Design review of the part built by this model. Coordinates are the model's own, in mm. A direction names the side the tool comes from. Give positions to 0.01 mm unless a question says otherwise; leave off trailing zeros. Order: outer loops, then holes, each group sorted by start corner. A loop starts at its lowest first (then second) coordinate and runs counter-clockwise, first axis right, second up. Notation, with made-up numbers: (14, 44.5) -> (64, 44.5) arc R12 ccw to (64, 66.5) -> close; hole circle Ø6 at (-1, 68). An arc over 180 degrees is marked (long way). Use a Markdown table: item, result. Add a question column.
```python
from build123d import *

# Parameters (mm, degrees)
BOSS_EXTRUDE1_DEPTH              = 9.525
TAP_DRILL_FOR_M3X0_5_TAP1_D      = 2.5
TAP_DRILL_FOR_M3X0_5_TAP2_D      = 2.5
TAP_DRILL_FOR_M3X0_5_TAP3_REACH  = 42.274
TAP_DRILL_FOR_M3X0_5_TAP3_BORE_R = 1.25
M3_CLEARANCE_HOLE1_REACH         = 42.274
M3_CLEARANCE_HOLE1_BORE_R        = 1.6


with BuildPart() as part:
    # Sketch1 → Boss-Extrude1 (new body)
    with BuildSketch(Plane(origin=(0, 0, 0), x_dir=(1, 0, 0), z_dir=(0, 1, 0))):
        with BuildLine():
            Line((-17.5, 17.5), (-5, 17.5))
            Line((-5, 17.5), (5, 17.5))
            Line((5, 17.5), (17.5, 17.5))
            Line((17.5, 17.5), (17.5, -17.5))
            Line((17.5, -17.5), (5, -17.5))
            Line((5, -17.5), (5, -8.660254038))
            ThreePointArc((5, -8.660254038), (10, 0), (5, 8.660254038))
            ThreePointArc((5, 8.660254038), (0, 10), (-5, 8.660254038))
            ThreePointArc((-5, 8.660254038), (-10, 0), (-5, -8.660254038))
            Line((-5, -8.660254038), (-5, -17.5))
            Line((-5, -17.5), (-17.5, -17.5))
            Line((-17.5, -17.5), (-17.5, 17.5))
        make_face()
    extrude(amount=BOSS_EXTRUDE1_DEPTH)

    # Tap Drill for M3x0.5 Tap1 (through all)
    with Locations(Plane(origin=(0, 9.525, 0), x_dir=(1, 0, 0), z_dir=(0, 1, 0))):
        with Locations((-15, 0)):
            Hole(TAP_DRILL_FOR_M3X0_5_TAP1_D / 2)

    # Tap Drill for M3x0.5 Tap2 (through all)
    with Locations(Plane(origin=(0, 9.525, 0), x_dir=(1, 0, 0), z_dir=(0, 1, 0))):
        with Locations((15, 0)):
            Hole(TAP_DRILL_FOR_M3X0_5_TAP2_D / 2)

    # Tap Drill for M3x0.5 Tap3 bore → Tap Drill for M3x0.5 Tap3 (cut, up to next)
    with BuildSketch(Plane(origin=(17.5, 0, 0), x_dir=(0, 0, -1), z_dir=(1, 0, 0)), mode=Mode.PRIVATE) as tap_drill_for_m3x0_5_tap3_sk1:
        with Locations((13.08015, 4.7625)):
            Circle(TAP_DRILL_FOR_M3X0_5_TAP3_BORE_R)
    tap_drill_for_m3x0_5_tap3_tool1 = extrude(tap_drill_for_m3x0_5_tap3_sk1.sketch, amount=-TAP_DRILL_FOR_M3X0_5_TAP3_REACH, mode=Mode.PRIVATE) & part.part
    # Tap Drill for M3x0.5 Tap3 bore → Tap Drill for M3x0.5 Tap3 (cut, up to next)
    with BuildSketch(Plane(origin=(17.5, 0, 0), x_dir=(0, 0, -1), z_dir=(1, 0, 0)), mode=Mode.PRIVATE) as tap_drill_for_m3x0_5_tap3_sk2:
        with Locations((-13.08015, 4.7625)):
            Circle(TAP_DRILL_FOR_M3X0_5_TAP3_BORE_R)
    tap_drill_for_m3x0_5_tap3_tool2 = extrude(tap_drill_for_m3x0_5_tap3_sk2.sketch, amount=-TAP_DRILL_FOR_M3X0_5_TAP3_REACH, mode=Mode.PRIVATE) & part.part
    add(tap_drill_for_m3x0_5_tap3_tool1.solids().sort_by_distance((17.5, 4.7625, -13.08015))[0], mode=Mode.SUBTRACT)
    add(tap_drill_for_m3x0_5_tap3_tool2.solids().sort_by_distance((17.5, 4.7625, 13.08015))[0], mode=Mode.SUBTRACT)

    # M3 Clearance Hole1 bore → M3 Clearance Hole1 (cut, up to next)
    with BuildSketch(Plane.ZY.offset(17.5), mode=Mode.PRIVATE) as m3_clearance_hole1_sk1:
        with Locations((-13.08015, 4.7625)):
            Circle(M3_CLEARANCE_HOLE1_BORE_R)
    m3_clearance_hole1_tool1 = extrude(m3_clearance_hole1_sk1.sketch, amount=-M3_CLEARANCE_HOLE1_REACH, mode=Mode.PRIVATE) & part.part
    # M3 Clearance Hole1 bore → M3 Clearance Hole1 (cut, up to next)
    with BuildSketch(Plane.ZY.offset(17.5), mode=Mode.PRIVATE) as m3_clearance_hole1_sk2:
        with Locations((13.08015, 4.7625)):
            Circle(M3_CLEARANCE_HOLE1_BORE_R)
    m3_clearance_hole1_tool2 = extrude(m3_clearance_hole1_sk2.sketch, amount=-M3_CLEARANCE_HOLE1_REACH, mode=Mode.PRIVATE) & part.part
    add(m3_clearance_hole1_tool1.solids().sort_by_distance((-17.5, 4.7625, -13.08015))[0], mode=Mode.SUBTRACT)
    add(m3_clearance_hole1_tool2.solids().sort_by_distance((-17.5, 4.7625, 13.08015))[0], mode=Mode.SUBTRACT)


solid = part.part
```
1) Add section C-C (x = -7). Give the boundary of the cut face in (y, z) (1 decimal), then the cut area to 3 significant figures.
2) Machinability: for faces 1 (the flat face through (-5, 5, 11)), 2 (the flat face through (17.5, 5, 0)), 3 (the cylindrical face through (-11.34, 4.83, 11.48)), which of the approach directions +Z, -Z, +X, -X, +Y, -Y give a long, thin tool a straight path to every point of the face, cutting with its end or side? Answer none if there is none.
3) Add section A-A (y = 7.5). Give the boundary of the cut face in (x, z), then the cut area to 3 significant figures.
4) For L1, parallel to Y at x = -5.5, z = 13 (1 decimal); L2, parallel to X at y = 5.5, z = 15.5; L3, parallel to X at y = 2, z = -0.5, list the stretches that pass through material, from the lowest coordinate up. Write a range as [from, to].
5) Add section B-B (z = 0). Give the boundary of the cut face in (x, y) (3 decimals).
6) Add section D-D (z = -6). Give the boundary of the cut face in (x, y) (3 decimals), then the cut area to 3 significant figures.
7) The part is to be moulded in two halves that separate along Z. For faces 4 (the flat face through (11, 5, 17.5)), 5 (the flat face through (-8, 9.525, -8)), 6 (the cylindrical face through (-0.25, 4.83, -14.68)), say which applies: +Z half, -Z half, draft (parallel to the pull), parting line (faces both ways), or undercut.
Worked answers:
| question | item | result |
|---|---|---|
| 1 | outline | (0, -17.5) -> (9.5, -17.5) -> (9.5, -7.1) -> (0, -7.1) -> close; (0, 7.1) -> (9.5, 7.1) -> (9.5, 17.5) -> (0, 17.5) -> close; hole circle Ø3.2 at (4.8, -13.1); hole circle Ø3.2 at (4.8, 13.1) |
| 1 | area | 181 mm^2 |
| 2 | face 1 | +Z, +Y, -Y |
| 2 | face 2 | +Z, -Z, +X, +Y, -Y |
| 2 | face 3 | -X |
| 3 | outline | (-17.5, -17.5) -> (17.5, -17.5) -> (17.5, 17.5) -> (5, 17.5) -> (5, 8.66) arc R10 cw (long way) to (-5, 8.66) -> (-5, 17.5) -> (-17.5, 17.5) -> close; hole circle Ø2.5 at (-15, 0); hole circle Ø2.5 at (15, 0) |
| 3 | area | 822 mm^2 |
| 4 | L1 | [0, 3.2], [6.4, 9.5] |
| 4 | L2 | [-17.5, -5], [5, 17.5] |
| 4 | L3 | [-17.5, -16.15], [-13.85, -9.99], [9.99, 13.85], [16.15, 17.5] |
| 5 | outline | (-17.5, 0) -> (-16.25, 0) -> (-16.25, 9.525) -> (-17.5, 9.525) -> close; (-13.75, 0) -> (-10, 0) -> (-10, 9.525) -> (-13.75, 9.525) -> close; (10, 0) -> (13.75, 0) -> (13.75, 9.525) -> (10, 9.525) -> close; (16.25, 0) -> (17.5, 0) -> (17.5, 9.525) -> (16.25, 9.525) -> close |
| 6 | outline | (-17.5, 0) -> (-8, 0) -> (-8, 9.525) -> (-17.5, 9.525) -> close; (8, 0) -> (17.5, 0) -> (17.5, 9.525) -> (8, 9.525) -> close |
| 6 | area | 181 mm^2 |
| 7 | face 4 | +Z half |
| 7 | face 5 | draft |
| 7 | face 6 | undercut |
